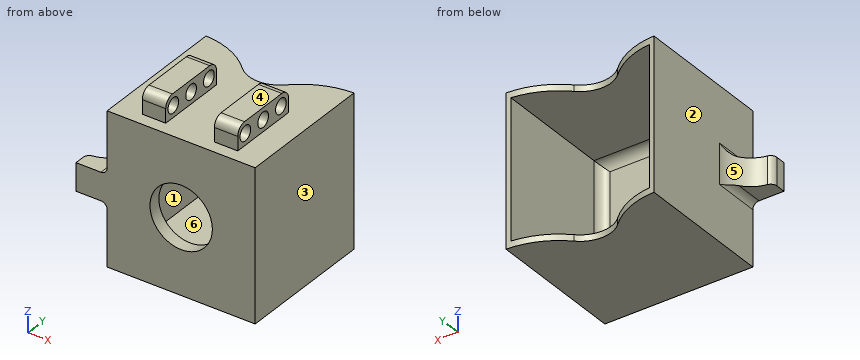
from build123d import *

# Parameters (mm, degrees)
SKETCH1_W               = 47.45
SKETCH1_H               = 48.45
BOSS_EXTRUDE1_DEPTH     = 44.45
SKETCH2_W               = 44.45
SKETCH2_H               = 44.45
CUT_EXTRUDE1_DEPTH      = 40.45
SKETCH3_W               = 7.5
SKETCH3_H               = 22.8
BOSS_EXTRUDE2_DEPTH     = 7.5
SKETCH4_R               = 2.4
CUT_EXTRUDE2_DEPTH      = 67.070738008
FILLET1_R               = 3
SKETCH5_W               = 8.878843291
SKETCH5_H               = 5
BOSS_EXTRUDE3_DEPTH     = 10
FILLET2_R               = 10
FILLET3_R               = 2
FILLET4_R               = 2
FILLET5_R               = 3
SKETCH6_R               = 10
CUT_EXTRUDE3_DEPTH      = 10
CUT_EXTRUDE5_DEPTH      = 83.857410319
CUT_EXTRUDE5_DEPTH_BACK = 83.857410319
FILLET6_R               = 25


# Some blends are built 0.0001 mm under size
with BuildPart() as part:
    # Sketch1 → Boss-Extrude1 (new body)
    with BuildSketch(Plane(origin=(0, 0, 0), x_dir=(1, 0, 0), z_dir=(0, 1, 0))):
        with Locations((-8.217167759, 5.212888782)):
            Rectangle(SKETCH1_W, SKETCH1_H)
    extrude(amount=BOSS_EXTRUDE1_DEPTH)

    # Sketch2 → Cut-Extrude1 (cut)
    with BuildSketch(Plane(origin=(0, 44.45, 0), x_dir=(1, 0, 0), z_dir=(0, 1, 0))):
        with Locations((-8.217167759, 5.212888782)):
            Rectangle(SKETCH2_W, SKETCH2_H)
    extrude(amount=-CUT_EXTRUDE1_DEPTH, mode=Mode.SUBTRACT)

    # Sketch3 → Boss-Extrude2 (add)
    with BuildSketch(Plane.XY.offset(19.012111218)):
        with Locations((-19.767167759, 15.4)):
            Rectangle(SKETCH3_W, SKETCH3_H)
        with Locations((3.332832241, 15.4)):
            Rectangle(SKETCH3_W, SKETCH3_H)
    extrude(amount=BOSS_EXTRUDE2_DEPTH)

    # Sketch4 → Cut-Extrude2 (cut, through all)
    with BuildSketch(Plane(origin=(7.082832241, 0, 0), x_dir=(0, 0, -1), z_dir=(1, 0, 0))):
        with Locations(Location((-22.762111218, 23.4, 0), (0, 0, 90))):
            Circle(SKETCH4_R)
        with Locations(Location((-22.762111218, 7.4, 0), (0, 0, 90))):
            Circle(SKETCH4_R)
        with Locations(Location((-22.762111218, 15.4, 0), (0, 0, 90))):
            Circle(SKETCH4_R)
    extrude(amount=-CUT_EXTRUDE2_DEPTH, mode=Mode.SUBTRACT)

    # Fillet1
    fillet1_edges = [part.edges().sort_by_distance(p)[0] for p in [
        (-19.767167759, 26.8, 26.512111218),
        (-19.767167759, 4, 26.512111218),
        (3.332832241, 26.8, 26.512111218),
        (3.332832241, 4, 26.512111218),
    ]]
    fillet(fillet1_edges, radius=FILLET1_R)

    # Sketch5 → Boss-Extrude3 (add)
    with BuildSketch(Plane.ZY.offset(31.942167759)):
        with Locations((-5.212888782, 2.5)):
            Rectangle(SKETCH5_W, SKETCH5_H)
    extrude(amount=BOSS_EXTRUDE3_DEPTH)

    # Fillet2
    fillet2_edges = [part.edges().sort_by_distance(p)[0] for p in [
        (-31.942167759, 5, -5.212888782),
    ]]
    fillet(fillet2_edges, radius=FILLET2_R - 0.0001)  # a hair under: the kernel refuses the full size

    # Fillet3
    fillet3_edges = [part.edges().sort_by_distance(p)[0] for p in [
        (-41.942167759, 5, -5.212888782),
    ]]
    fillet(fillet3_edges, radius=FILLET3_R)

    # Fillet4
    fillet4_edges = [part.edges().sort_by_distance(p)[0] for p in [
        (-31.942167759, 7.49995, -9.652310427),
        (-31.942167759, 7.49995, -0.773467136),
    ]]
    fillet(fillet4_edges, radius=FILLET4_R)

    # Fillet5
    fillet5_edges = [part.edges().sort_by_distance(p)[0] for p in [
        (-30.442167759, 4, -5.212888782),
        (-8.217167759, 4, -27.437888782),
        (14.007832241, 4, -5.212888782),
        (-8.217167759, 4, 17.012111218),
    ]]
    fillet(fillet5_edges, radius=FILLET5_R)

    # Sketch6 → Cut-Extrude3 (cut)
    with BuildSketch(Plane(origin=(0, 4, 0), x_dir=(1, 0, 0), z_dir=(0, 1, 0))):
        with Locations(Location((-8.217167759, 5.212888782, 0), (0, 0, 270))):
            Circle(SKETCH6_R)
    extrude(amount=-CUT_EXTRUDE3_DEPTH, mode=Mode.SUBTRACT)

    # Sketch7 → Cut-Extrude5 (cut, two sides: drawn at the far end of the back side and taken through both)
    with BuildSketch(Plane(origin=(0, 0, -29.437888782), x_dir=(-1, 0, 0), z_dir=(0, 0, -1)).offset(-CUT_EXTRUDE5_DEPTH_BACK)):
        with BuildLine():
            Line((18.217167759, 179.152496248), (18.217167759, 44.45))
            ThreePointArc((18.217167759, 44.45), (8.217167759, 34.45), (-1.782832241, 44.45))
            Line((-1.782832241, 44.45), (-1.782832241, 179.152496248))
            Line((-1.782832241, 179.152496248), (-1.782832241, 448.557488745))
            Line((-1.782832241, 448.557488745), (18.217167759, 448.557488745))
            Line((18.217167759, 448.557488745), (18.217167759, 179.152496248))
        make_face()
    extrude(amount=CUT_EXTRUDE5_DEPTH + CUT_EXTRUDE5_DEPTH_BACK, mode=Mode.SUBTRACT)

    # Fillet6
    # the kernel refuses this fillet: 25 mm, written as the material it takes off along each edge
    with BuildSketch(Plane(origin=(1.782832241, 44.45, -17.300388782), x_dir=(1, 0, 0), z_dir=(0, 0, 1)), Plane(origin=(1.782832241, 44.45, -63.750388782), x_dir=(1, 0, 0), z_dir=(0, 0, 1))) as fillet6_piece_1:
        with BuildLine():
            CenterArc((14.507389357, -24.987754339), FILLET6_R, 91.793397152, 42.650547852)
            Line((-2.997888755, -7.139358382), (-3.347994317, -6.782390463))
            ThreePointArc((-3.347994317, -6.782390463), (-1.240888915, -3.678039288), (-0.5, 0))
            Line((-0.5, 0), (0, 0.5))
            ThreePointArc((0, 0.5), (6.8625, 0.5), (13.709352213, 0.499755087))
            Line((13.709352213, 0.499755087), (13.725, 0))
        make_face()
    extrude(amount=70.625, mode=Mode.SUBTRACT)
    with BuildSketch(Plane(origin=(-18.217167759, 44.45, -17.300388782), x_dir=(-1, 0, 0), z_dir=(0, 0, 1)), Plane(origin=(-18.217167759, 44.45, -63.750388782), x_dir=(-1, 0, 0), z_dir=(0, 0, 1))) as fillet6_piece_2:
        with BuildLine():
            CenterArc((14.507389357, 24.987754339), FILLET6_R, 225.556054997, 42.650547852)
            Line((-2.997888755, 7.139358382), (-3.347994317, 6.782390463))
            ThreePointArc((-3.347994317, 6.782390463), (-1.240888915, 3.678039288), (-0.5, 0))
            Line((-0.5, 0), (0, -0.5))
            ThreePointArc((0, -0.5), (6.8625, -0.5), (13.709352213, -0.499755087))
            Line((13.709352213, -0.499755087), (13.725, 0))
        make_face()
    extrude(amount=70.625, mode=Mode.SUBTRACT)


solid = part.part
Part model, mm, in its own coordinate system. Face numbers are marked on the shaded views. A direction names the side the tool comes from. Give positions to 0.01 mm unless a question says otherwise; leave off trailing zeros. Order: outer loops, then holes, each group sorted by start corner. A loop starts at its lowest first (then second) coordinate and runs counter-clockwise, first axis right, second up. Notation, with made-up numbers: (68.5, -8) - (85.5, -8) arc R22 ccw to (85.5, 20) - close; hole circle Ø6 at (30, -17). An arc over 180 degrees is marked (long way). Use a Markdown table: item, result.
1) Saw through at A-A on y = 22.5. List the corners of the cut face in (x, z).
Checked values:
| item | result |
|---|---|
| outline | (-31.94, -29.44) - (15.51, -29.44) - (15.51, 19.01) - (7.08, 19.01) - (7.08, 20.54) - (-0.42, 20.54) - (-0.42, 19.01) - (-16.02, 19.01) - (-16.02, 20.54) - (-23.52, 20.54) - (-23.52, 19.01) - (-31.94, 19.01) - close; (-23.52, 24.99) - (-16.02, 24.99) - (-16.02, 26.51) - (-23.52, 26.51) - close; (-0.42, 24.99) - (7.08, 24.99) - (7.08, 26.51) - (-0.42, 26.51) - close; hole (-30.44, -27.44) - (14.01, -27.44) - (14.01, 17.01) - (-30.44, 17.01) - close |
2) Flat gauge pins, fed straight in: P1, Ø2, axis at x = -20.5, z = 22, coming from the +Y side; P2, Ø8, axis at y = 12, z = 22.5, coming from the -X side; P3, Ø19, axis at x = -11, z = 2.5, coming from the +Y side. Where does each tip first touch, or does it go through?
Checked values:
| item | result |
|---|---|
| P1 | y = 26.8 |
| P2 | x = -31.94 |
| P3 | y = 4 |
3) Saw through at D-D on y = 41. List the corners of the cut face in (x, z).
Checked values:
| item | result |
|---|---|
| outline | (-31.94, -29.44) - (-20.03, -29.44) - (-20.03, -27.44) - (-30.44, -27.44) - (-30.44, 17.01) - (-20.03, 17.01) - (-20.03, 19.01) - (-31.94, 19.01) - close; (3.6, -29.44) - (15.51, -29.44) - (15.51, 19.01) - (3.6, 19.01) - (3.6, 17.01) - (14.01, 17.01) - (14.01, -27.44) - (3.6, -27.44) - close |
4) Two-plate mould, pull along Z, no slides. Class the marked faces 4, 5 and 6: +Z half, -Z half, draft (parallel to the pull), parting line (faces both ways), or undercut.
Checked values:
| item | result |
|---|---|
| face 4 | +Z half |
| face 5 | draft |
| face 6 | undercut |
5) Saw through at C-C on z = -18. List the corners of the cut face in (x, y), plus the area to 3 significant figures.
Checked values:
| item | result |
|---|---|
| outline | (-31.94, 0) - (15.51, 0) - (15.51, 44.45) arc R25 ccw to (14.01, 44.36) - (14.01, 7) arc R3 cw to (11.01, 4) - (-27.44, 4) arc R3 cw to (-30.44, 7) - (-30.44, 44.36) arc R25 ccw to (-31.94, 44.45) - close |
| area | 315 mm² |
6) Probe L1, parallel to Z at x = 4.5, y = 7.4; L2, parallel to Z at x = 12.5, y = 29; L3, parallel to X at y = 36.5, z = 1. List the from-to ranges inside material, lowest first. Write a range as from..to.
Checked values:
| item | result |
|---|---|
| L1 | -29.44..-27.44, 17.01..20.36, 25.16..26.51 |
| L2 | -29.44..-27.44, 17.01..19.01 |
| L3 | -31.94..-30.44, 14.01..15.51 |
7) 3-axis set-ups, long thin cutter, end or side, ignore diameter. For the marked faces 1, 2 and 3: which of +Z, -Z, +X, -X, +Y, -Y reach the whole face in a straight line?
Checked values:
| item | result |
|---|---|
| face 1 | +Y |
| face 2 | -X, +Y |
| face 3 | +Z, -Z, +X, +Y, -Y |
8) Saw through at B-B on x = -17. List the corners of the cut face in (y, z), plus the area to 3 significant figures.
Checked values:
| item | result |
|---|---|
| outline | (0, -29.44) - (38.9, -29.44) - (38.9, -27.44) - (7, -27.44) arc R3 cw to (4, -24.44) - (4, -9.99) - (0, -9.99) - close; (0, -0.43) - (4, -0.43) - (4, 14.01) arc R3 cw to (7, 17.01) - (38.9, 17.01) - (38.9, 19.01) - (26.8, 19.01) - (26.8, 23.51) arc R3 ccw to (23.8, 26.51) - (7, 26.51) arc R3 ccw to (4, 23.51) - (4, 19.01) - (0, 19.01) - close; hole circle Ø4.8 at (7.4, 22.76); hole circle Ø4.8 at (15.4, 22.76); hole circle Ø4.8 at (23.4, 22.76) |
| area | 412 mm² |
